from build123d import *

# Parameters (mm, degrees)
SKETCH1_R           = 6.2
BOSS_EXTRUDE1_DEPTH = 5.4
SKETCH2_R           = 3
BOSS_EXTRUDE3_DEPTH = 102.1
BOSS_EXTRUDE4_START = 5.4
SKETCH4_R           = 6.2
BOSS_EXTRUDE4_DEPTH = 5.4


with BuildPart() as part:
    # Sketch1 → Boss-Extrude1 (new body)
    with BuildSketch(Plane.XY):
        with BuildLine():
            Line((0, 0), (-149.578947368, 0))
            ThreePointArc((-149.578947368, 0), (-174.878947368, -25.3), (-149.578947368, -50.6))
            Line((-149.578947368, -50.6), (130.421052632, -50.6))
            ThreePointArc((130.421052632, -50.6), (155.721052632, -25.3), (130.421052632, 0))
            Line((130.421052632, 0), (0, 0))
        make_face()
        with Locations(Location((130.421052632, -25.3, 0), (0, 0, 180))):
            Circle(SKETCH1_R, mode=Mode.SUBTRACT)
    extrude(amount=BOSS_EXTRUDE1_DEPTH)

    # Sketch2 → Boss-Extrude3 (add)
    with BuildSketch(Plane(origin=(0, 0, 0), x_dir=(-1, 0, 0), z_dir=(0, 0, -1))):
        with Locations(Location((-68.985809966, -25.3, 0), (0, 0, 180))):
            Circle(SKETCH2_R)
    extrude(amount=BOSS_EXTRUDE3_DEPTH)

    # Sketch4 → Boss-Extrude4 (add)
    with BuildSketch(Plane(origin=(0, 0, -102.1), x_dir=(-1, 0, 0), z_dir=(0, 0, -1)).offset(BOSS_EXTRUDE4_START)):
        with BuildLine():
            Line((-130.421052632, 0), (149.578947368, 0))
            ThreePointArc((149.578947368, 0), (174.878947368, -25.3), (149.578947368, -50.6))
            Line((149.578947368, -50.6), (-130.421052632, -50.6))
            ThreePointArc((-130.421052632, -50.6), (-155.721052632, -25.3), (-130.421052632, 0))
        make_face()
        with Locations((-130.421052632, -25.3)):
            Circle(SKETCH4_R, mode=Mode.SUBTRACT)
    extrude(amount=-BOSS_EXTRUDE4_DEPTH)


solid = part.part
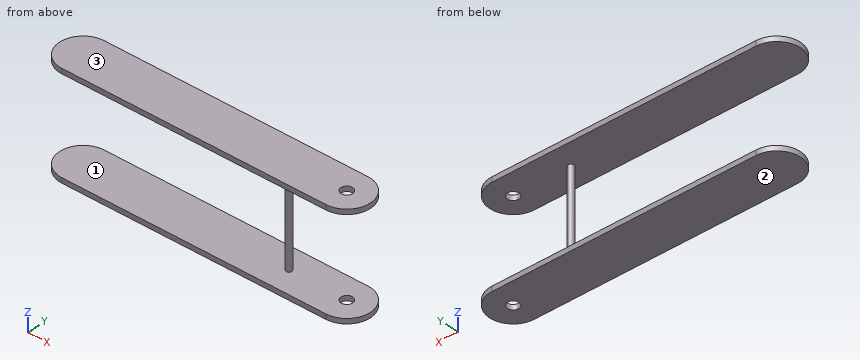
Here's how the part is built. I have some questions about the finished solid (model axes, mm). Face numbers are marked on the shaded views. Round coordinates to 2 decimals unless told otherwise and drop trailing zeros. Write each loop counter-clockwise with the first axis right and the second up, starting at its lowest first coordinate (ties: lowest second). Pieces come first, ordered by that corner, then holes.
1. I need wall thicknesses on L1, parallel to Z at x = 105.5, y = -10; L2, parallel to X at y = -25, z = -106; L3, parallel to Y at x = 70, z = -83.5. Which ranges of each line are inside material? Lowest first, please.
2. Suppose I cut it at B-B (x = -34.5). List the corners of the cut face in (y, z) for me, and give its area (3 significant figures).
3. Suppose I cut it at C-C (y = -10). List the corners of the cut face in (x, z) for me.
4. Suppose I cut it at D-D (z = -21). List the corners of the cut face in (x, y) for me, and give its area (3 significant figures).
5. Suppose I cut it at A-A (y = -25.3). List the corners of the cut face in (x, z) for me.
6. Will these pins go through, and if not, where does the flat tip stop? pin 1 Ø7.5 at (x, y) = (130.42, -25.3) entering from -Z; pin 2 Ø12 at (y, z) = (-34, -16) entering from +X; pin 3 Ø12 at (y, z) = (-28, -38) entering from -X.
7. If we mould it in two halves opening along Z, with no side actions, what happens to the marked faces 1, 2 and 3? For each: released by +Z, released by -Z, zero draft, split by the parting line, or undercut.
Answer sheet:
1. L1: z = -107.5 to -102.1, 0 to 5.4
1. L2: x = -174.88 to 124.23, 136.61 to 155.72
1. L3: y = -28.12 to -22.48
2. outline: (-50.6, -107.5) - (0, -107.5) - (0, -102.1) - (-50.6, -102.1) - close; (-50.6, 0) - (0, 0) - (0, 5.4) - (-50.6, 5.4) - close
2. area: 546 mm2
3. outline: (-169.73, -107.5) - (150.57, -107.5) - (150.57, -102.1) - (-169.73, -102.1) - close; (-169.73, 0) - (150.57, 0) - (150.57, 5.4) - (-169.73, 5.4) - close
4. outline: circle Ø6 at (68.99, -25.3)
4. area: 28.3 mm2
5. outline: (-174.88, -107.5) - (124.22, -107.5) - (124.22, -102.1) - (71.99, -102.1) - (71.99, 0) - (124.22, 0) - (124.22, 5.4) - (-174.88, 5.4) - (-174.88, 0) - (65.99, 0) - (65.99, -102.1) - (-174.88, -102.1) - close; (136.62, -107.5) - (155.72, -107.5) - (155.72, -102.1) - (136.62, -102.1) - close; (136.62, 0) - (155.72, 0) - (155.72, 5.4) - (136.62, 5.4) - close
6. pin 1: passes through
6. pin 2: stops at x = 70.29
6. pin 3: stops at x = 65.99
7. face 1: undercut
7. face 2: released by -Z
7. face 3: released by +Z
